For this review, take the finished solid that the model builds, in its own axes (mm). Face numbers are marked on the shaded views. A direction names the side the tool comes from. Coordinates: 2 decimals unless noted, no trailing zeros. Write each loop counter-clockwise with the first axis right and the second up, starting at its lowest first coordinate (ties: lowest second). Pieces come first, ordered by that corner, then holes.
1) For the marked faces 4, 5 and 6, list the 3-axis set-ups (+Z, -Z, +X, -X, +Y, -Y) from which the entire face can be reached by the end or side of a thin tool; tool diameter is ignored.
2) We need section A-A on z = 9. Write out the cut boundary in (x, y) (3 decimals).
3) Mouldability with a two-part tool opening along Y and no side actions: class the marked faces 1, 2 and 3 as pulls with the +Y half, pulls with the -Y half, needs draft (parallel to the pull), parting line crosses it, or undercut.
4) To check wall thickness, follow line 1 along Y through (x, z) = (15.24, -2.95); line 2 along X through (y, z) = (26, -3.5); line 3 along X through (y, z) = (21, 10.5). State the ranges of each line that lie inside material, in increasing order.
5) Insertion check: P1, Ø1.3, axis at x = -56.81, y = 37.83, coming from the -Z side; P2, Ø1.2, axis at x = 15.24, y = 18.19, coming from the +Z side; P3, Ø1, axis at x = 1, z = -2.5, coming from the -Y side. Each pin has a flat end and moves straight along its axis. Give the tip position at first contact, or say it passes through.
6) We need section B-B on x = -18. Write out the cut boundary in (y, z).
from build123d import *

# Parameters (mm, degrees)
BOSS_EXTRUDE1_DEPTH = 15.24
CUT_EXTRUDE1_DEPTH  = 24.492240162
SKETCH3_W           = 139.7
SKETCH3_H           = 44
BOSS_EXTRUDE2_DEPTH = 9.3472
FILLET1_R           = 6.35
SKETCH6_R           = 6.1595
CUT_EXTRUDE2_DEPTH  = 93.183607262
SKETCH7_R           = 0.9652
CUT_EXTRUDE3_DEPTH  = 5.588
SKETCH8_R           = 0.80645
CUT_EXTRUDE4_DEPTH  = 5.08
SKETCH9_R           = 14.175
SKETCH9_R_2         = 11
BOSS_EXTRUDE5_DEPTH = 6.985
FILLET2_R           = 2.54


with BuildPart() as part:
    # Sketch1 → Boss-Extrude1 (new body)
    with BuildSketch(Plane(origin=(0, 0, 0), x_dir=(0, 0, -1), z_dir=(1, 0, 0))):
        Polygon((-4.6736, 0), (-4.6736, 5.08), (4.6736, 5.08), (4.6736, 0), (4.6736, -15.24), (1.6256, -15.24), (1.6256, 0), (-1.6256, 0), (-1.6256, -15.24), (-4.6736, -15.24), align=None)
    extrude(amount=-BOSS_EXTRUDE1_DEPTH)

    # Sketch2 → Cut-Extrude1 (cut, through all)
    with BuildSketch(Plane.XY.offset(4.6736)):
        with BuildLine():
            ThreePointArc((-5.08, -7.62), (-5.823948776, -5.823948776), (-7.62, -5.08))
            Line((-7.62, -5.08), (-7.62, -10.16))
            ThreePointArc((-7.62, -10.16), (-5.823948776, -9.416051224), (-5.08, -7.62))
        make_face()
        with BuildLine():
            Line((-7.62, -10.16), (-7.62, -5.08))
            ThreePointArc((-7.62, -5.08), (-10.16, -7.62), (-7.62, -10.16))
        make_face()
        with BuildLine():
            ThreePointArc((-7.62, -15.24), (-13.008153673, -13.008153673), (-15.24, -7.62))
            Line((-15.24, -7.62), (-15.24, -15.24))
            Line((-15.24, -15.24), (-7.62, -15.24))
        make_face()
        with BuildLine():
            Line((0, -15.24), (0, -7.62))
            ThreePointArc((0, -7.62), (-2.231846327, -13.008153673), (-7.62, -15.24))
            Line((-7.62, -15.24), (0, -15.24))
        make_face()
    extrude(amount=-CUT_EXTRUDE1_DEPTH, mode=Mode.SUBTRACT)

    # Sketch3 → Boss-Extrude2 (add)
    with BuildSketch(Plane.XY.offset(4.6736)):
        with Locations((-7.62, 27.08)):
            Rectangle(SKETCH3_W, SKETCH3_H)
    extrude(amount=-BOSS_EXTRUDE2_DEPTH)

    # Fillet1
    fillet1_edges = [part.edges().sort_by_distance(p)[0] for p in [
        (62.23, 5.08, 0),
        (62.23, 49.08, 0),
        (-77.47, 49.08, 0),
        (-77.47, 5.08, 0),
    ]]
    fillet(fillet1_edges, radius=FILLET1_R)

    # Sketch6 → Cut-Extrude2 (cut, through all)
    with BuildSketch(Plane.XY.offset(4.6736)):
        with Locations((-56.809999918, 29.08)):
            Circle(SKETCH6_R)
        with Locations((41.569999918, 29.08)):
            Circle(SKETCH6_R)
    extrude(amount=-CUT_EXTRUDE2_DEPTH, mode=Mode.SUBTRACT)

    # Sketch7 → Cut-Extrude3 (cut)
    with BuildSketch(Plane(origin=(0, 0, -4.6736), x_dir=(-1, 0, 0), z_dir=(0, 0, -1))):
        with Locations((30.48, 35.97)):
            Circle(SKETCH7_R)
        with Locations((-15.24, 35.97)):
            Circle(SKETCH7_R)
        with Locations((30.48, 18.19)):
            Circle(SKETCH7_R)
        with Locations((-15.24, 18.19)):
            Circle(SKETCH7_R)
        with Locations((7.62, 7.649)):
            Circle(SKETCH7_R)
        with Locations((7.62, 46.511)):
            Circle(SKETCH7_R)
    extrude(amount=-CUT_EXTRUDE3_DEPTH, mode=Mode.SUBTRACT)

    # Sketch8 → Cut-Extrude4 (cut)
    with BuildSketch(Plane(origin=(0, 0, -4.6736), x_dir=(-1, 0, 0), z_dir=(0, 0, -1))):
        with Locations((-41.57, 37.83)):
            Circle(SKETCH8_R)
        with Locations((-41.57, 9.83)):
            Circle(SKETCH8_R)
        with Locations((56.81, 37.83)):
            Circle(SKETCH8_R)
        with Locations((56.81, 9.83)):
            Circle(SKETCH8_R)
    extrude(amount=-CUT_EXTRUDE4_DEPTH, mode=Mode.SUBTRACT)

    # Sketch9 → Boss-Extrude5 (add)
    with BuildSketch(Plane.XY.offset(4.6736)):
        with Locations((-56.81, 29.08)):
            Circle(SKETCH9_R)
        with Locations(Location((-56.81, 29.08, 0), (0, 0, 270))):
            Circle(SKETCH9_R_2, mode=Mode.SUBTRACT)
        with Locations((41.57, 29.08)):
            Circle(SKETCH9_R)
        with Locations(Location((41.57, 29.08, 0), (0, 0, 270))):
            Circle(SKETCH9_R_2, mode=Mode.SUBTRACT)
    extrude(amount=BOSS_EXTRUDE5_DEPTH)

    # Fillet2
    fillet2_edges = [part.edges().sort_by_distance(p)[0] for p in [
        (-70.985, 29.08, 4.6736),
        (27.395, 29.08, 4.6736),
    ]]
    fillet(fillet2_edges, radius=FILLET2_R)


solid = part.part
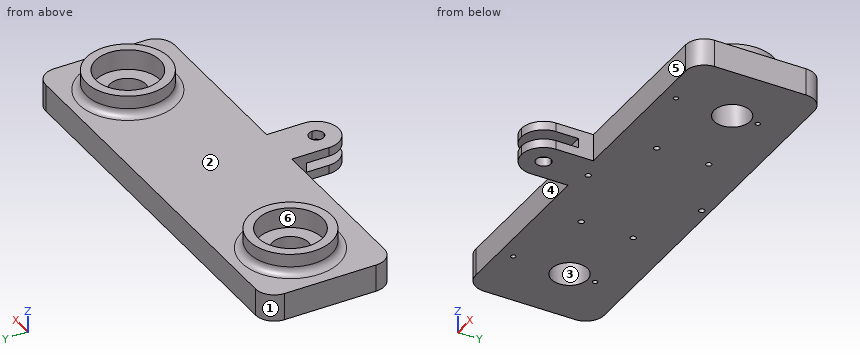
Result:
1. face 4: +Z, -Z, -X, -Y
1. face 5: +Z, -Z, +X, -Y
1. face 6: +Z
2. outline: circle Ø28.35 at (-56.81, 29.08); circle Ø28.35 at (41.57, 29.08); hole circle Ø22 at (-56.81, 29.08); hole circle Ø22 at (41.57, 29.08)
3. face 1: pulls with the +Y half
3. face 2: needs draft
3. face 3: undercut
4. line 1: y = 5.08 to 17.22, 19.16 to 35, 36.94 to 49.08
4. line 2: x = -77.47 to -62.14, -51.48 to 36.24, 46.9 to 62.23
4. line 3: x = -68.46 to -64.27, -49.35 to -45.16, 29.92 to 34.11, 49.03 to 53.22
5. P1: stops at z = 0.41
5. P2: stops at z = 4.67
5. P3: stops at y = 5.08
6. outline: (5.08, -4.67) - (49.08, -4.67) - (49.08, 4.67) - (5.08, 4.67) - close
